Read the model definition and answer for the solid it produces. Units are mm, in the model's axes. A direction names the side the tool comes from. Round coordinates to 2 decimals unless told otherwise and drop trailing zeros. Order: outer loops, then holes, each group sorted by start corner. A loop starts at its lowest first (then second) coordinate and runs counter-clockwise, first axis right, second up. Notation, with made-up numbers: (1.5, 77.25) -> (32.5, 77.25) arc R23 cw to (32.5, 110.25) -> close; hole circle Ø10 at (-34.5, -32). An arc over 180 degrees is marked (long way). Answer as a JSON object with one key per item and string values. Group by question number.
Item 1: Section D-D, the plane y = -33 is taken. Write down the section's boundary in (x, z).
Item 2: The mould has two halves that part along Z. Classify faces 1 (the cylindrical face through (232.9, -20.3, 11.2)), 2 (the flat face through (243.826, -29, 148)), 3 (the flat face through (92, -10, 20)): pulls with the +Z half, pulls with the -Z half, needs draft (parallel to the pull), parting line crosses it, or undercut.
Item 3: Section B-B, the plane y = -7.5 is taken. Write down the section's boundary in (x, z), plus the area to 3 significant figures.
Item 4: For faces 4 (the flat face through (92, -11, 0)), 5 (the flat face through (229, -20, 162)), 6 (the flat face through (77, -20, 10)), determine the directions among +Z, -Z, +X, -X, +Y, -Y from which every point of the face is accessible in a straight line to the end or side of a thin tool.
Item 5: Consider probe 1 along Z at (x, y) = (73.5, -8.5); probe 2 along X at (y, z) = (-33, 140). Determine where each line is inside the solid, lowest interval first. Write a range as from..to.
Item 6: Given P1, Ø6, axis at x = 115.5, z = 7.5, coming from the -Y side; P2, Ø10, axis at y = -33, z = 197.5, coming from the -X side; P3, Ø16, axis at x = 49, y = -10.5, coming from the +Z side, each flat-ended and moving along its own axis, determine where each tip first touches the part or whether it passes through.
Item 7: Section C-C, the plane z = 128.5 is taken. Write down the section's boundary in (x, y).
Item 8: Section A-A, the plane x = 93.5 is taken. Write down the section's boundary in (y, z).
from build123d import *

# Parameters (mm, degrees)
F0_W     = 300
F0_H     = 20
F1_DEPTH = 20
F2_R     = 5.1542561855
F3_DEPTH = 20.001
F4_W     = 30
F4_H     = 300
F5_DEPTH = 20
F6_R     = 5.1542561855
F7_DEPTH = 25


with BuildPart() as f1:
    # F0 (on Front) → F1 (new body)
    with BuildSketch(Plane.XZ):
        with Locations((93.8255012718, 10)):
            Rectangle(F0_W, F0_H)
    extrude(amount=F1_DEPTH)

    # F2 (on face) → F3 (cut, through all)
    with BuildSketch(Plane.XZ.offset(20)):
        with Locations((227.9840409756, 9.651648812)):
            Circle(F2_R)
    extrude(amount=-F3_DEPTH, mode=Mode.SUBTRACT)

    # F4 (on face) → F5 (join)
    with BuildSketch(Plane.XZ.offset(20)):
        with Locations((228.8255012718, 150)):
            Rectangle(F4_W, F4_H)
    extrude(amount=F5_DEPTH)

    # F6 (on face) → F7 (cut)
    with BuildSketch(Plane.XZ.offset(40)):
        with Locations((227.9840409756, 9.651648812)):
            Circle(F6_R)
    extrude(amount=-F7_DEPTH, mode=Mode.SUBTRACT)


solid = f1.part
Values found:
{
 "1": {"outline": "(213.83, 0) -> (243.83, 0) -> (243.83, 300) -> (213.83, 300) -> close; hole circle Ø10.31 at (227.98, 9.65)"},
 "2": {"face 1": "undercut", "face 2": "needs draft", "face 3": "pulls with the +Z half"},
 "3": {"outline": "(-56.17, 0) -> (243.83, 0) -> (243.83, 20) -> (-56.17, 20) -> close; hole circle Ø10.31 at (227.98, 9.65)", "area": "5,920 mm2"},
 "4": {"face 4": "-Z, +X, -X, +Y, -Y", "face 5": "+Z, +X, -X, +Y", "face 6": "+Z, -Z, -X, -Y"},
 "5": {"probe 1": "0..20", "probe 2": "213.83..243.83"},
 "6": {"P1": "y = -20", "P2": "x = 213.83", "P3": "z = 20"},
 "7": {"outline": "(213.83, -40) -> (243.83, -40) -> (243.83, -20) -> (213.83, -20) -> close"},
 "8": {"outline": "(-20, 0) -> (0, 0) -> (0, 20) -> (-20, 20) -> close"}
}
